Geometry check sheet. Reference: the model listing, model coordinates, mm. A direction names the side the tool comes from. Round coordinates to 2 decimals unless told otherwise and drop trailing zeros. Write each loop counter-clockwise with the first axis right and the second up, starting at its lowest first coordinate (ties: lowest second). Pieces come first, ordered by that corner, then holes.
Item 1: Depth check by flat-ended pin: P1, Ø1, axis at x = 24, y = -15, coming from the +Z side; P2, Ø1.5, axis at x = 8.5, y = -15.5, coming from the -Z side; P3, Ø1.5, axis at x = 10.5, z = 3, coming from the +Y side; P4, Ø0.9, axis at x = 1.5, y = -24, coming from the -Z side. Enter the tip coordinate at first touch or a pass-through.
Item 2: Scan lines: probe 1 along Y at (x, z) = (1.15, 12); probe 2 along Z at (x, y) = (23, -22); probe 3 along X at (y, z) = (-16, 10). Record each from-to range of solid material in increasing order.
Item 3: Cross-section at C-C (y = -12). Enter the section's corners in (x, z).
Item 4: Cross-section at B-B (z = 12). Enter the section's corners in (x, y), then the cut area to 3 significant figures.
Item 5: Cross-section at A-A (x = 4). Enter the section's corners in (y, z).
Item 6: Cross-section at D-D (x = 19.5). Enter the section's corners in (y, z).
Item 7: Access from +Z, -Z, +X, -X, +Y, -Y to the whole of each face (thin tool, end or side, straight path). Record for faces 5 (the face through (47.5, -11.9, 1.5)), 6 (the face through (36, -20, 3)), 7 (the face through (10, -21, 1)).
Item 8: Draft check along Y on faces 1 (the face through (1, 3, 9)), 2 (the face through (41, -36.634, 1)), 3 (the face through (4, -31.849, 3)), 4 (the face through (25, -19, 0)). Enter one of: pulls with the +Y half, pulls with the -Y half, needs draft (parallel to the pull), parting line crosses it, or undercut.
Autodesk Inventor part; units mm, degrees
ref_plane "YZ Plane" through (0, 0, 0) normal (1, 0, 0) x (0, 1, 0)
ref_plane "XZ Plane" through (0, 0, 0) normal (0, 1, 0) x (-1, 0, 0)
ref_plane "XY Plane" through (0, 0, 0) normal (0, 0, 1) x (1, 0, 0)
sketch "Sketch1" plane through (0, 0, 0) normal (0, 0, 1) x (1, 0, 0)
  line L0 (0, 0) -> (50, 0)
  line L1 (50, 0) -> (50, -40)
  line L2 (50, -40) -> (0, -40)
  line L3 (0, -40) -> (0, 0)
  dimension "d0" = 50
  dimension "d1" = 40
extrude "Extrusion1" add sketch "Sketch1" along normal blind 3
sketch "Sketch2" plane through (0, 0, 3) normal (0, 0, 1) x (1, 0, 0)
  line L0 (0, -40) -> (50, -40)
  line L1 (0, 0) -> (3, 0)
  line L2 (3, 0) -> (3, -40)
  line L3 (3, -40) -> (0, -40)
  line L4 (0, -40) -> (0, 0)
  dimension "d4" = 3
extrude "Extrusion2" add sketch "Sketch2" along normal blind 15
sketch "Sketch3" plane through (0, 0, 0) normal (0, 1, 0) x (1, 0, 0)
  line L0 (0, 0) -> (3, 0)
  line L1 (3, 0) -> (3, -18)
  line L2 (3, -18) -> (0, -18)
  line L3 (0, -18) -> (0, 0)
extrude "Extrusion3" add sketch "Sketch3" along normal blind 3
sketch "Sketch4" plane through (0, 0, 0) normal (0, 0, -1) x (-1, 0, 0)
  line L0 (0, -40) -> (0, 3)
  line L1 (-3, 0) -> (-3, 3)
  line L2 (-3, 0) -> (-3, -11)
  line L3 (0, -11) -> (-10, -11)
  line L4 (-10, -11) -> (-10, -31.8493)
  line L5 (-10, -31.8493) -> (0, -31.8493)
  point P0 (0, 0)
  dimension "d9" = 11
  dimension "d10" = 10
extrude "Extrusion4" cut sketch "Sketch4" against normal blind 8
sketch "Sketch6" plane through (0, -40, 0) normal (-1, 0, 0) x (0, 0, 1)
  circle A0 centre (12, 38) radius 2
  point P0 (0, 40)
  dimension "d17" = 4
extrude "Extrusion6" cut sketch "Sketch6" against normal through all
sketch "Sketch7" plane through (0, -40, 0) normal (-1, 0, 0) x (0, 0, 1)
  circle A0 centre (12, 7) radius 2
  point P0 (0, 40)
  dimension "d21" = 4
extrude "Extrusion7" cut sketch "Sketch7" against normal through all
sketch "Sketch8" plane through (0, 0, 0) normal (0, 0, -1) x (-1, 0, 0)
  line L0 (-45, -12) -> (-37, -12) construction
  line L1 (-45, -14.5) -> (-37, -14.5)
  line L2 (-37, -9.5) -> (-45, -9.5)
  arc A0 (-45, -9.5) -> (-45, -14.5) centre (-45, -12) ccw
  arc A1 (-37, -14.5) -> (-37, -9.5) centre (-37, -12) ccw
  point P0 (0, 0)
  point P1 (-41, -12)
  dimension "d27" = 8
  dimension "d28" = 5
extrude "Extrusion8" cut sketch "Sketch8" against normal through all
sketch "Sketch9" plane through (0, 0, 0) normal (0, 0, -1) x (-1, 0, 0)
  line L0 (-37, -14.5) -> (-45, -14.5)
  line L1 (-45, -34.1343) -> (-37, -34.1343) construction
  line L2 (-45, -36.6343) -> (-37, -36.6343)
  line L3 (-37, -31.6343) -> (-45, -31.6343)
  arc A0 (-45, -31.6343) -> (-45, -36.6343) centre (-45, -34.1343) ccw
  arc A1 (-37, -36.6343) -> (-37, -31.6343) centre (-37, -34.1343) ccw
  point P0 (0, 0)
  point P1 (-41, -34.1343)
  dimension "d31" = 8
  dimension "d32" = 5
extrude "Extrusion9" cut sketch "Sketch9" against normal through all
sketch "Sketch10" plane through (0, 0, 3) normal (0, 0, 1) x (1, 0, 0)
  line L0 (11.4775, -1.7089) -> (32.8001, -1.7089)
  line L1 (32.8001, -1.7089) -> (32.8001, -38.2911)
  line L2 (32.8001, -38.2911) -> (11.4775, -38.2911)
  line L3 (11.4775, -38.2911) -> (11.4775, -1.7089)
  point P0 (0, 0)
extrude "Extrusion10" cut sketch "Sketch10" against normal blind 1
chamfer "Chamfer1" distance 3 angle 45 1 edges at (3, -35.9246, 3)
chamfer "Chamfer2" distance 3 angle 45 1 edges at (3, -5.5, 3)
properties part number "bart z endstop bracket v9"
Resolved:
1. P1: stops at z = 2
1. P2: passes through
1. P3: stops at y = 0
1. P4: stops at z = 8
2. probe 1: y = -40 to -35, -31 to -4, 0 to 3
2. probe 2: z = 0 to 2
2. probe 3: x = 0 to 3
3. outline: (0, 8) - (3, 8) - (3, 18) - (0, 18) - close; (10, 0) - (34.5, 0) - (34.5, 3) - (32.8, 3) - (32.8, 2) - (11.48, 2) - (11.48, 3) - (10, 3) - close; (47.5, 0) - (50, 0) - (50, 3) - (47.5, 3) - close
4. outline: (0, -40) - (3, -40) - (3, -35) - (0, -35) - close; (0, -31) - (3, -31) - (3, -4) - (0, -4) - close; (0, 0) - (3, 0) - (3, 3) - (0, 3) - close
4. area: 105 mm2
5. outline: (-40, 0) - (-31.85, 0) - (-31.85, 5) - (-40, 5) - close; (-11, 0) - (0, 0) - (0, 5) - (-11, 5) - close
6. outline: (-40, 0) - (0, 0) - (0, 3) - (-1.71, 3) - (-1.71, 2) - (-38.29, 2) - (-38.29, 3) - (-40, 3) - close
7. face 5: +Z, -Z
7. face 6: +Z, +X, +Y, -Y
7. face 7: +Z, -Z, -X
8. face 1: pulls with the +Y half
8. face 2: undercut
8. face 3: undercut
8. face 4: needs draft
